from build123d import *

# Parameters (mm, degrees)
F0_R     = 15.5
F0_R_2   = 12.5
F1_DEPTH = 15
F0_R_3   = 26
F0_R_4   = 22.5
F3_R     = 4.6577592735
F4_DEPTH = 11


with BuildPart() as f1:
    # F0 (on Front) → F1 (new body)
    with BuildSketch(Plane.XZ):
        Circle(F0_R)
        Circle(F0_R_2, mode=Mode.SUBTRACT)
    extrude(amount=-F1_DEPTH)



with BuildPart() as f1b:
    # F0 (on Front) → F1, piece 2 (new body)
    with BuildSketch(Plane.XZ):
        Circle(F0_R_3)
        Circle(F0_R_4, mode=Mode.SUBTRACT)
    extrude(amount=-F1_DEPTH)


with BuildPart() as f1_1:
    add(f1.part)

    add(f1b.part)  # F4 merges F1b
    # F3 (on offset) → F4 (join)
    with BuildSketch(Plane.XZ.offset(-2)):
        with Locations((0, 19)):
            Circle(F3_R)
        with Locations((-11.1679197936, 15.3713228931)):
            Circle(F3_R)
        with Locations((-18.0700738096, 5.8713228931)):
            Circle(F3_R)
        with Locations((-18.0700738096, -5.8713228931)):
            Circle(F3_R)
        with Locations((-11.1679197936, -15.3713228931)):
            Circle(F3_R)
        with Locations((0, -19)):
            Circle(F3_R)
        with Locations((11.1679197936, -15.3713228931)):
            Circle(F3_R)
        with Locations((18.0700738096, -5.8713228931)):
            Circle(F3_R)
        with Locations((18.0700738096, 5.8713228931)):
            Circle(F3_R)
        with Locations((11.1679197936, 15.3713228931)):
            Circle(F3_R)
    extrude(amount=-F4_DEPTH)


solid = f1_1.part
Build history of the part. All positions in model axes, mm. A direction names the side the tool comes from. Coordinates: 2 decimals unless noted, no trailing zeros. Order: outer loops, then holes, each group sorted by start corner. A loop starts at its lowest first (then second) coordinate and runs counter-clockwise, first axis right, second up. Notation, with made-up numbers: (-30.75, 30) - (-16.75, 30) arc R35 cw to (-16.75, 69) - close; hole circle Ø3 at (72, 55). An arc over 180 degrees is marked (long way). Write item = value, one per line. Start each with the question number.
1) Two-plate mould, pull along X, no slides. Class faces 1 (the face through (16.33, 7.42, 10.19)), 2 (the face through (1, 15, 13)), 3 (the face through (-4.647, 7.423, 18.677)): pulls with the +X half, pulls with the -X half, needs draft (parallel to the pull), parting line crosses it, or undercut.
2) Wall check: line 1 along Z through (x, y) = (0, 9); line 2 along Z through (x, y) = (-8, 6.25); line 3 along Z through (x, y) = (-6, 6). Give the ranges that are in metal, low to high. Write a range as from..to.
3) Saw through at C-C on z = 0. Write the cut outline in (x, y), then the cut area to 3 significant figures.
4) Saw through at A-A on x = 0. Write the cut outline in (y, z).
5) Flat gauge pins, fed straight in: pin 1 Ø1.5 at (y, z) = (10.5, 14) entering from +X; pin 2 Ø4 at (x, y) = (15, 6) entering from +Z; pin 3 Ø2 at (x, z) = (10, 16) entering from -Y. Where does each tip first touch, or does it go through?
6) 3-axis set-ups, long thin cutter, end or side, ignore diameter. For faces 4 (the face through (0, 13, 19)), 5 (the face through (-11.7, 15, 19.4)), 6 (the face through (18, 2, 6)): which of +Z, -Z, +X, -X, +Y, -Y reach the whole face in a straight line?
7) Saw through at D-D on y = 1. Write the cut outline in (x, z).
8) Saw through at B-B on z = 6. Write the cut outline in (x, y).
From the geometry:
q1.face_1 = undercut
q1.face_2 = needs draft
q1.face_3 = undercut
q2.line_1 = -26..-12.5, 12.5..26
q2.line_2 = -24.74..-21.03, -18.79..-9.6, 9.6..18.79, 21.03..24.74
q2.line_3 = -25.3..-21.69, -14.29..-10.97, 10.97..14.29, 21.69..25.3
q3.outline = (-26, 0) - (-22.5, 0) - (-22.5, 15) - (-26, 15) - close; (-15.5, 0) - (-12.5, 0) - (-12.5, 15) - (-15.5, 15) - close; (12.5, 0) - (15.5, 0) - (15.5, 15) - (12.5, 15) - close; (22.5, 0) - (26, 0) - (26, 15) - (22.5, 15) - close
q3.area = 195 mm^2
q4.outline = (0, -26) - (15, -26) - (15, -22.5) - (13, -22.5) - (13, -15.5) - (15, -15.5) - (15, -12.5) - (0, -12.5) - (0, -15.5) - (2, -15.5) - (2, -22.5) - (0, -22.5) - close; (0, 12.5) - (15, 12.5) - (15, 15.5) - (13, 15.5) - (13, 22.5) - (15, 22.5) - (15, 26) - (0, 26) - (0, 22.5) - (2, 22.5) - (2, 15.5) - (0, 15.5) - close
q5.pin_1 = 22.37
q5.pin_2 = 22.52
q5.pin_3 = 2
q6.face_4 = +Y
q6.face_5 = +Z, -Z, +X, -X, +Y
q6.face_6 = -Y
q7.outline = circle Ø52 at (0, 0); circle Ø31 at (0, 0); hole circle Ø45 at (0, 0); hole circle Ø25 at (0, 0)
q8.outline = (-25.3, 0) - (-21.69, 0) - (-21.69, 2) - (-14.29, 2) - (-14.29, 0) - (-10.97, 0) - (-10.97, 15) - (-14.29, 15) - (-14.29, 13) - (-21.69, 13) - (-21.69, 15) - (-25.3, 15) - close; (10.97, 0) - (14.29, 0) - (14.29, 2) - (21.69, 2) - (21.69, 0) - (25.3, 0) - (25.3, 15) - (21.69, 15) - (21.69, 13) - (14.29, 13) - (14.29, 15) - (10.97, 15) - close
